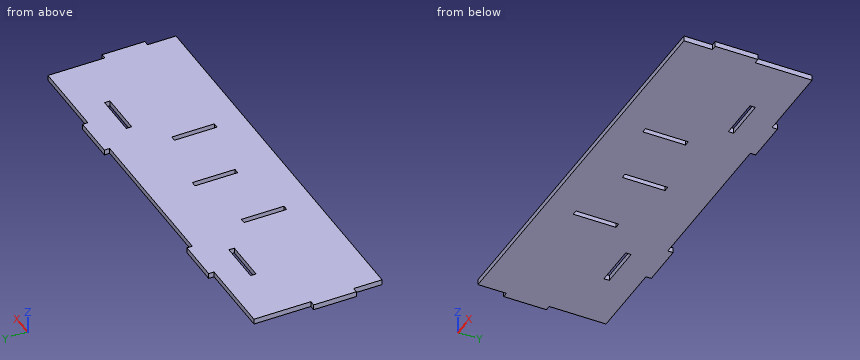
```python
from build123d import *

# Parameters (mm, degrees)
F0_W     = 19.05
F0_H     = 152.4
F0_W_2   = 152.4
F0_H_2   = 19.05
F1_DEPTH = 19.05


with BuildPart() as f1:
    # F0 (on Top) → F1 (new body)
    with BuildSketch(Plane.XY):
        Polygon((-441.325, 0), (-720.725, 0), (-720.725, -203.2), (-720.725, -355.6), (-720.725, -457.2), (720.725, -457.2), (720.725, -355.6), (720.725, -203.2), (720.725, 0), (441.325, 0), (288.925, 0), (-288.925, 0), align=None)
        with Locations((-243.416667, -279.4)):
            Rectangle(F0_W, F0_H, mode=Mode.SUBTRACT)
        with Locations((243.416667, -279.4)):
            Rectangle(F0_W, F0_H, mode=Mode.SUBTRACT)
        with Locations((0, -228.6)):
            Rectangle(F0_W, F0_H, mode=Mode.SUBTRACT)
        with Locations((-434.975, -104.775)):
            Rectangle(F0_W_2, F0_H_2, mode=Mode.SUBTRACT)
        with Locations((434.975, -104.775)):
            Rectangle(F0_W_2, F0_H_2, mode=Mode.SUBTRACT)
        with Locations((-365.125, 9.525)):
            Rectangle(F0_W_2, F0_H_2)
        with Locations((365.125, 9.525)):
            Rectangle(F0_W_2, F0_H_2)
        with Locations((730.25, -279.4)):
            Rectangle(F0_W, F0_H)
        with Locations((-730.25, -279.4)):
            Rectangle(F0_W, F0_H)
    extrude(amount=F1_DEPTH)


solid = f1.part
```
CAD build for the part. Positions are in the model's coordinates, mm. Coordinates: 2 decimals unless noted, no trailing zeros. Order: outer loops, then holes, each group sorted by start corner. A loop starts at its lowest first (then second) coordinate and runs counter-clockwise, first axis right, second up. Notation, with made-up numbers: (52, 79) -> (88, 79) arc R22 ccw to (88, 88) -> close; hole circle Ø4 at (4.5, 19.5). An arc over 180 degrees is marked (long way). Use one line per item in the form item = value. Start each with the question number.
1) Band-saw the part on C-C on z = 7. State how many separate pieces and enclosed holes the cut face has, then the cut area to 3 significant figures.
2) Drill centre lines: L1, parallel to X at y = -253, z = 4.5 (3 decimals); L2, parallel to Y at x = -237.5, z = 17; L3, parallel to Y at x = -371, z = 3.5. Where is each one in solid material? Low to high. Write a range as [from, to].
3) Band-saw the part on B-B on y = -169.5. Give the cut face in (x, z) (3 decimals).
4) Band-saw the part on A-A on x = -424.5. Give the cut face in (y, z).
5) Band-saw the part on D-D on x = -91. Give the cut face in (y, z).
6) Drop flat-ended pins along their axis: pin 1 (4 mm diameter, centred on x = -462, z = 3, fed in from +Y); pin 2 (1.5 mm diameter, centred on y = -152, z = 9, fed in from +X) (3 decimals); pin 3 (5.5 mm diameter, centred on y = -136.5, z = 7.5, fed in from -X) (3 decimals). Give the stop position or say it passes through.
Entries:
q1.separate_pieces = 1
q1.enclosed_holes = 5
q1.area = 656,000 mm2
q2.L1 = [-739.775, -252.942], [-233.892, -9.525], [9.525, 233.892], [252.942, 739.775]
q2.L2 = [-457.2, -355.6], [-203.2, 0]
q2.L3 = [-457.2, -114.3], [-95.25, 19.05]
q3.outline = (-720.725, 0) -> (-9.525, 0) -> (-9.525, 19.05) -> (-720.725, 19.05) -> close; (9.525, 0) -> (720.725, 0) -> (720.725, 19.05) -> (9.525, 19.05) -> close
q4.outline = (-457.2, 0) -> (-114.3, 0) -> (-114.3, 19.05) -> (-457.2, 19.05) -> close; (-95.25, 0) -> (19.05, 0) -> (19.05, 19.05) -> (-95.25, 19.05) -> close
q5.outline = (-457.2, 0) -> (0, 0) -> (0, 19.05) -> (-457.2, 19.05) -> close
q6.pin_1 = 0
q6.pin_2 = 720.725
q6.pin_3 = -720.725
